Design review of the part built by this model. Coordinates are the model's own, in mm. A direction names the side the tool comes from. Coordinates: 2 decimals unless noted, no trailing zeros. Write each loop counter-clockwise with the first axis right and the second up, starting at its lowest first coordinate (ties: lowest second). Pieces come first, ordered by that corner, then holes.
Q1. Clearance check with flat-ended pins moving along their axes: pin 1 Ø4 at (x, y) = (-62.74, 0) entering from -Z; pin 2 Ø7.5 at (x, y) = (1, 91) entering from -Z; pin 3 Ø5 at (y, z) = (-76, 2.5) entering from -X; pin 4 Ø1.5 at (x, z) = (-42, 7.5) entering from +Y. State where each tip first meets the part, or that it passes through.
Q2. Add section B-B, the plane x = -44. Give the boundary of the cut face in (y, z).
Q3. Add section A-A, the plane z = 5.25. Give the boundary of the cut face in (x, y).
Q4. The part is to be moulded in two halves that separate along Y. For faces 6 (the face through (-5, -100, 5)), 7 (the face through (-65.935, 1.006, 0.813)), 8 (the face through (-27, 1, 10)), say which applies: +Y half, -Y half, draft (parallel to the pull), parting line (faces both ways), or undercut.
Q5. To check wall thickness, follow probe 1 along Y at (x, z) = (-26.25, 5); probe 2 along Y at (x, z) = (0, 0.6); probe 3 along Y at (x, z) = (-62.74, 3.75). State the ranges of each line that lie inside material, in increasing order.
Q6. Machinability: for faces 1 (the face through (0.44, 93.32, 0.81)), 2 (the face through (-61.04, 0.07, 5.77)), 3 (the face through (-21.25, 80, 5)), 4 (the face through (-27, 1, 0)), 5 (the face through (-21.25, -80, 5)), which of the approach directions +Z, -Z, +X, -X, +Y, -Y give a long, thin tool a straight path to every point of the face, cutting with its end or side? Answer none if there is none.
from build123d import *

# Parameters (mm, degrees)
BOSS_EXTRUDE1_DEPTH             = 10
SKETCH4_R                       = 1.7
CUT_EXTRUDE3_DEPTH              = 15
CBORE_FOR_M3_SBHCS1_D           = 3.4
CBORE_FOR_M3_SBHCS1_DEPTH       = 3.15
CBORE_FOR_M3_SBHCS1_CBORE_D     = 6.7
CBORE_FOR_M3_SBHCS1_CBORE_DEPTH = 1.65
CBORE_FOR_M3_SBHCS1_TIP         = 1.021463052
CBORE_FOR_M3_SBHCS2_D           = 3.4
CBORE_FOR_M3_SBHCS2_DEPTH       = 3.15
CBORE_FOR_M3_SBHCS2_CBORE_D     = 6.7
CBORE_FOR_M3_SBHCS2_CBORE_DEPTH = 1.65
CBORE_FOR_M3_SBHCS2_TIP         = 1.021463052
SKETCH7_W                       = 65
SKETCH7_H                       = 120
BOSS_EXTRUDE2_DEPTH             = 10
SKETCH9_W                       = 10
SKETCH9_H                       = 120
BOSS_EXTRUDE3_DEPTH             = 12
SKETCH10_W                      = 65
SKETCH10_H                      = 120
BOSS_EXTRUDE4_DEPTH             = 7
SKETCH11_R                      = 11
BOSS_EXTRUDE5_DEPTH             = 12
SKETCH13_W                      = 65
SKETCH13_H                      = 120
CUT_EXTRUDE4_DEPTH              = 19
SKETCH14_R                      = 1.7
CUT_EXTRUDE5_DEPTH              = 15
CBORE_FOR_M3_SBHCS3_D           = 3.4
CBORE_FOR_M3_SBHCS3_DEPTH       = 3.15
CBORE_FOR_M3_SBHCS3_CBORE_D     = 6.7
CBORE_FOR_M3_SBHCS3_CBORE_DEPTH = 1.65
CBORE_FOR_M3_SBHCS3_TIP         = 1.021463052
SKETCH17_R                      = 1.7
CUT_EXTRUDE6_DEPTH              = 10
CBORE_FOR_M3_SBHCS4_D           = 3.4
CBORE_FOR_M3_SBHCS4_DEPTH       = 3.15
CBORE_FOR_M3_SBHCS4_CBORE_D     = 6.7
CBORE_FOR_M3_SBHCS4_CBORE_DEPTH = 1.65
CBORE_FOR_M3_SBHCS4_TIP         = 1.021463052


with BuildPart() as part:
    # Sketch1 → Boss-Extrude1 (new body)
    with BuildSketch(Plane(origin=(0, 0, 0), x_dir=(0, 1, 0), z_dir=(0, 0, 1))):
        Polygon((-100, 11.25), (-100, 21.25), (100, 21.25), (100, 11.25), (100, -11.25), (-100, -11.25), align=None)
    extrude(amount=BOSS_EXTRUDE1_DEPTH)

    # Sketch4 → Cut-Extrude3 (cut)
    with BuildSketch(Plane.XY.offset(10)):
        with Locations((0, 90)):
            Circle(SKETCH4_R)
        with Locations((0, -90)):
            Circle(SKETCH4_R)
    extrude(amount=-CUT_EXTRUDE3_DEPTH, mode=Mode.SUBTRACT)

    # CBORE for M3 SBHCS1
    with Locations(Plane(origin=(0, 90, 0), x_dir=(-1, 0, 0), z_dir=(0, 0, -1))):
        with Locations((0, 0)):
            CounterBoreHole(CBORE_FOR_M3_SBHCS1_D / 2, CBORE_FOR_M3_SBHCS1_CBORE_D / 2, CBORE_FOR_M3_SBHCS1_CBORE_DEPTH, depth=CBORE_FOR_M3_SBHCS1_DEPTH)
            with Locations((0, 0, -(CBORE_FOR_M3_SBHCS1_DEPTH + CBORE_FOR_M3_SBHCS1_TIP / 2))):  # 118° drill point
                Cone(0, CBORE_FOR_M3_SBHCS1_D / 2, CBORE_FOR_M3_SBHCS1_TIP, mode=Mode.SUBTRACT)

    # CBORE for M3 SBHCS2
    with Locations(Plane(origin=(0, -90, 0), x_dir=(-1, 0, 0), z_dir=(0, 0, -1))):
        with Locations((0, 0)):
            CounterBoreHole(CBORE_FOR_M3_SBHCS2_D / 2, CBORE_FOR_M3_SBHCS2_CBORE_D / 2, CBORE_FOR_M3_SBHCS2_CBORE_DEPTH, depth=CBORE_FOR_M3_SBHCS2_DEPTH)
            with Locations((0, 0, -(CBORE_FOR_M3_SBHCS2_DEPTH + CBORE_FOR_M3_SBHCS2_TIP / 2))):  # 118° drill point
                Cone(0, CBORE_FOR_M3_SBHCS2_D / 2, CBORE_FOR_M3_SBHCS2_TIP, mode=Mode.SUBTRACT)

    # Sketch7 → Boss-Extrude2 (add)
    with BuildSketch(Plane(origin=(0, 0, 0), x_dir=(1, 0, 0), z_dir=(0, 0, -1))):
        with Locations((-53.75, 0)):
            Rectangle(SKETCH7_W, SKETCH7_H)
    extrude(amount=-BOSS_EXTRUDE2_DEPTH)

    # Sketch9 → Boss-Extrude3 (add)
    with BuildSketch(Plane.XY.offset(10)):
        with Locations((-26.25, 0)):
            Rectangle(SKETCH9_W, SKETCH9_H)
    extrude(amount=BOSS_EXTRUDE3_DEPTH)

    # Sketch10 → Boss-Extrude4 (add)
    with BuildSketch(Plane.XY.offset(22)):
        with Locations((-53.75, 0)):
            Rectangle(SKETCH10_W, SKETCH10_H)
    extrude(amount=BOSS_EXTRUDE4_DEPTH)

    # Sketch11 → Boss-Extrude5 (add)
    with BuildSketch(Plane(origin=(0, 0, 22), x_dir=(1, 0, 0), z_dir=(0, 0, -1))):
        with Locations(Location((-62.74, 0, 0), (0, 0, 180))):
            Circle(SKETCH11_R)
    extrude(amount=BOSS_EXTRUDE5_DEPTH)

    # Sketch13 → Cut-Extrude4 (cut)
    with BuildSketch(Plane.XY.offset(29)):
        with Locations((-53.75, 0)):
            Rectangle(SKETCH13_W, SKETCH13_H)
    extrude(amount=-CUT_EXTRUDE4_DEPTH, mode=Mode.SUBTRACT)

    # Sketch14 → Cut-Extrude5 (cut)
    with BuildSketch(Plane(origin=(0, 0, 0), x_dir=(1, 0, 0), z_dir=(0, 0, -1))):
        with Locations(Location((-26.25, 50, 0), (0, 0, 180))):
            Circle(SKETCH14_R)
        with Locations(Location((-26.25, -50, 0), (0, 0, 180))):
            Circle(SKETCH14_R)
    extrude(amount=-CUT_EXTRUDE5_DEPTH, mode=Mode.SUBTRACT)

    # CBORE for M3 SBHCS3
    with Locations(Plane(origin=(-26.25, -50, 0), x_dir=(-1, 0, 0), z_dir=(0, 0, -1))):
        with Locations((0, 0), (0, 100)):
            CounterBoreHole(CBORE_FOR_M3_SBHCS3_D / 2, CBORE_FOR_M3_SBHCS3_CBORE_D / 2, CBORE_FOR_M3_SBHCS3_CBORE_DEPTH, depth=CBORE_FOR_M3_SBHCS3_DEPTH)
            with Locations((0, 0, -(CBORE_FOR_M3_SBHCS3_DEPTH + CBORE_FOR_M3_SBHCS3_TIP / 2))):  # 118° drill point
                Cone(0, CBORE_FOR_M3_SBHCS3_D / 2, CBORE_FOR_M3_SBHCS3_TIP, mode=Mode.SUBTRACT)

    # Sketch17 → Cut-Extrude6 (cut)
    with BuildSketch(Plane(origin=(0, 0, 0), x_dir=(1, 0, 0), z_dir=(0, 0, -1))):
        with Locations(Location((-62.74, 0, 0), (0, 0, 180))):
            Circle(SKETCH17_R)
    extrude(amount=-CUT_EXTRUDE6_DEPTH, mode=Mode.SUBTRACT)

    # CBORE for M3 SBHCS4
    with Locations(Plane(origin=(-62.74, 0, 0), x_dir=(-1, 0, 0), z_dir=(0, 0, -1))):
        with Locations((0, 0)):
            CounterBoreHole(CBORE_FOR_M3_SBHCS4_D / 2, CBORE_FOR_M3_SBHCS4_CBORE_D / 2, CBORE_FOR_M3_SBHCS4_CBORE_DEPTH, depth=CBORE_FOR_M3_SBHCS4_DEPTH)
            with Locations((0, 0, -(CBORE_FOR_M3_SBHCS4_DEPTH + CBORE_FOR_M3_SBHCS4_TIP / 2))):  # 118° drill point
                Cone(0, CBORE_FOR_M3_SBHCS4_D / 2, CBORE_FOR_M3_SBHCS4_TIP, mode=Mode.SUBTRACT)


solid = part.part
Here are the results:
1. pin 1: stops at z = 1.65
1. pin 2: stops at z = 0
1. pin 3: stops at x = -21.25
1. pin 4: stops at y = 60
2. outline: (-60, 0) - (60, 0) - (60, 10) - (-60, 10) - close
3. outline: (-86.25, -60) - (-21.25, -60) - (-21.25, -100) - (11.25, -100) - (11.25, 100) - (-21.25, 100) - (-21.25, 60) - (-86.25, 60) - close; hole circle Ø3.4 at (-62.74, 0); hole circle Ø3.4 at (-26.25, -50); hole circle Ø3.4 at (-26.25, 50); hole circle Ø3.4 at (0, -90); hole circle Ø3.4 at (0, 90)
4. face 6: -Y half
4. face 7: undercut
4. face 8: draft
5. probe 1: y = -60 to -51.7, -48.3 to 48.3, 51.7 to 60
5. probe 2: y = -100 to -93.35, -86.65 to 86.65, 93.35 to 100
5. probe 3: y = -60 to -1.7, 1.7 to 60
6. face 1: -Z
6. face 2: +Z, -Z
6. face 3: +Z, -Z, -X, +Y
6. face 4: -Z, +X, -X, +Y, -Y
6. face 5: +Z, -Z, -X, -Y
